Could you check a few things on this drawing? It's one solid part, dimensions in mm from its lowest x, y, z. Round coordinates to 2 decimals unless told otherwise and drop trailing zeros. Write each loop counter-clockwise with the first axis right and the second up, starting at its lowest first coordinate (ties: lowest second). Pieces come first, ordered by that corner, then holes. Notation, with made-up numbers: (39.5, 74) -> (51.5, 74) arc R21 cw to (51.5, 94) -> close; hole circle Ø6 at (48.5, 31). An arc over 180 degrees is marked (long way). Put each result on its own line as item: value. Start each with the question number.
1) I want a section at D-D, the plane x = 39. List the corners of the cut face in (y, z) for me, then the cut area to 3 significant figures.
2) If I drill on line 1 along X through (y, z) = (5, 2.9); line 2 along Y through (x, z) = (30, 2.15); line 3 along Y through (x, z) = (29, 3.25), over which ranges is the centre line in solid material (lowest first)? Write a range as [from, to].
3) I want a section at B-B, the plane x = 75. List the corners of the cut face in (y, z) for me.
4) I want a section at A-A, the plane y = 5. List the corners of the cut face in (x, z) for me, then the cut area to 3 significant figures.
5) I want a section at C-C, the plane z = 4.1. List the corners of the cut face in (x, y) for me.
6) Will this pin go through, and if not, where does the flat tip stop? P1, Ø1, axis at y = 119.5, z = 2, coming from the -X side.
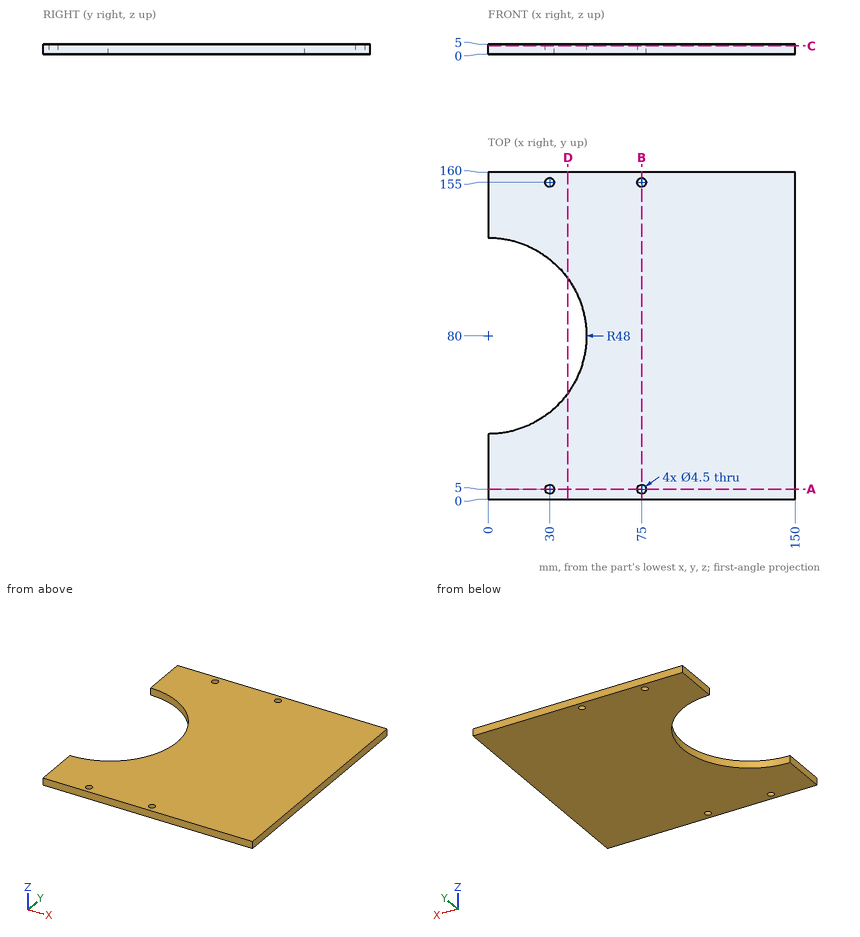
Findings:
1. outline: (0, 0) -> (52.02, 0) -> (52.02, 5) -> (0, 5) -> close; (107.98, 0) -> (160, 0) -> (160, 5) -> (107.98, 5) -> close
1. area: 520 mm2
2. line 1: x = [0, 27.75], [32.25, 72.75], [77.25, 150]
2. line 2: y = [0, 2.75], [7.25, 42.53], [117.47, 152.75], [157.25, 160]
2. line 3: y = [0, 2.98], [7.02, 41.75], [118.25, 152.98], [157.02, 160]
3. outline: (0, 0) -> (2.75, 0) -> (2.75, 5) -> (0, 5) -> close; (7.25, 0) -> (152.75, 0) -> (152.75, 5) -> (7.25, 5) -> close; (157.25, 0) -> (160, 0) -> (160, 5) -> (157.25, 5) -> close
4. outline: (0, 0) -> (27.75, 0) -> (27.75, 5) -> (0, 5) -> close; (32.25, 0) -> (72.75, 0) -> (72.75, 5) -> (32.25, 5) -> close; (77.25, 0) -> (150, 0) -> (150, 5) -> (77.25, 5) -> close
4. area: 705 mm2
5. outline: (0, 0) -> (150, 0) -> (150, 160) -> (0, 160) -> (0, 128) arc R48 cw to (0, 32) -> close; hole circle Ø4.5 at (30, 5); hole circle Ø4.5 at (30, 155); hole circle Ø4.5 at (75, 5); hole circle Ø4.5 at (75, 155)
6. P1: stops at x = 26.53
